Geometry: final body of the model. Coordinates: model frame, mm. Face numbers are marked on the shaded views. A direction names the side the tool comes from. Give positions to 0.01 mm unless a question says otherwise; leave off trailing zeros. Write each loop counter-clockwise with the first axis right and the second up, starting at its lowest first coordinate (ties: lowest second). Pieces come first, ordered by that corner, then holes.
from build123d import *

# Parameters (mm, degrees)
F0_W     = 198.306992
F0_H     = 131.550192
F1_DEPTH = 76.2
F2_W     = 175.236628
F2_H     = 111.424976
F3_DEPTH = 76.201
F4_R     = 17.935486
F5_DEPTH = 198.307993
F6_W     = 76.328561
F6_H     = 10.062608
F7_DEPTH = 38.1


with BuildPart() as f1:
    # F0 (on Top) → F1 (new body)
    with BuildSketch(Plane.XY):
        Rectangle(F0_W, F0_H)
    extrude(amount=F1_DEPTH)

    # F2 (on face) → F3 (cut, through all)
    with BuildSketch(Plane.XY.offset(76.2)):
        Rectangle(F2_W, F2_H)
    extrude(amount=-F3_DEPTH, mode=Mode.SUBTRACT)

    # F4 (on face) → F5 (cut, through all)
    with BuildSketch(Plane.YZ.offset(99.153496)):
        with Locations((0, 38.1)):
            Circle(F4_R)
    extrude(amount=-F5_DEPTH, mode=Mode.SUBTRACT)

    # F6 (on face) → F7 (cut)
    with BuildSketch(Plane.XY.offset(76.2)):
        with Locations((-0.859004, 60.743792)):
            Rectangle(F6_W, F6_H)
        with Locations((-0.859004, -60.743792)):
            Rectangle(F6_W, F6_H)
    extrude(amount=-F7_DEPTH, mode=Mode.SUBTRACT)


solid = f1.part
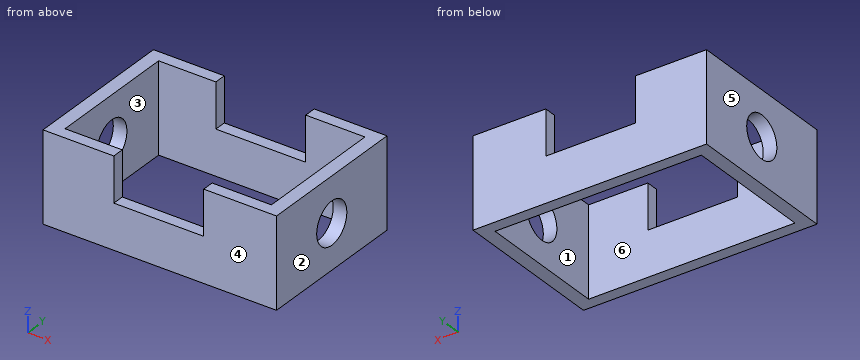
Q1. Section D-D on z = 16. Output: boundary loops of the cut face in (x, y), plus the area to 3 significant figures.
Filled sheet:
outline: (-99.15, -65.78) - (99.15, -65.78) - (99.15, 65.78) - (-99.15, 65.78) - close; hole (-87.62, -55.71) - (87.62, -55.71) - (87.62, 55.71) - (-87.62, 55.71) - close
area: 6,560 mm2
Q2. Pull-direction query (Y, two-part tool) for the marked faces 3, 4, 5 and 6; classes: released by +Y, released by -Y, zero draft, split by the parting line, or undercut.
Filled sheet:
face 3: undercut
face 4: released by -Y
face 5: zero draft
face 6: undercut
Q3. Pin query (flat end, axial travel): P1, Ø5, axis at x = -13.5, y = 60, coming from the +Z side. Return the tip coordinate at first contact, or that it passes through.
Filled sheet:
P1: stops at z = 38.1
Q4. Section A-A on x = 22.5. Output: boundary loops of the cut face in (y, z), plus the area to 3 significant figures.
Filled sheet:
outline: (-65.78, 0) - (-55.71, 0) - (-55.71, 38.1) - (-65.78, 38.1) - close; (55.71, 0) - (65.78, 0) - (65.78, 38.1) - (55.71, 38.1) - close
area: 767 mm2
Q5. Access query for the marked faces 1 and 2. Directions: +Z, -Z, +X, -X, +Y, -Y. A direction counts if a zero-diameter tool reaches every point of the face in a straight line with its end or side. Return the directions, or none.
Filled sheet:
face 1: +Z, -Z
face 2: +Z, -Z, +X, +Y, -Y
Q6. Section C-C on y = 0. Output: boundary loops of the cut face in (x, z).
Filled sheet:
outline: (-99.15, 0) - (-87.62, 0) - (-87.62, 20.16) - (-99.15, 20.16) - close; (-99.15, 56.04) - (-87.62, 56.04) - (-87.62, 76.2) - (-99.15, 76.2) - close; (87.62, 0) - (99.15, 0) - (99.15, 20.16) - (87.62, 20.16) - close; (87.62, 56.04) - (99.15, 56.04) - (99.15, 76.2) - (87.62, 76.2) - close
Q7. Section B-B on z = 63. Output: boundary loops of the cut face in (x, y).
Filled sheet:
outline: (-99.15, -65.78) - (-39.02, -65.78) - (-39.02, -55.71) - (-87.62, -55.71) - (-87.62, 55.71) - (-39.02, 55.71) - (-39.02, 65.78) - (-99.15, 65.78) - close; (37.31, -65.78) - (99.15, -65.78) - (99.15, 65.78) - (37.31, 65.78) - (37.31, 55.71) - (87.62, 55.71) - (87.62, -55.71) - (37.31, -55.71) - close
Q8. Ray query, line 1 along X through (y, z) = (0, 63); line 2 along Y through (x, z) = (49, 12.5); line 3 along Z through (x, y) = (95.25, 0). Return the intervals inside material, ascending.
Filled sheet:
line 1: x = -99.15 to -87.62, 87.62 to 99.15
line 2: y = -65.78 to -55.71, 55.71 to 65.78
line 3: z = 0 to 20.16, 56.04 to 76.2
